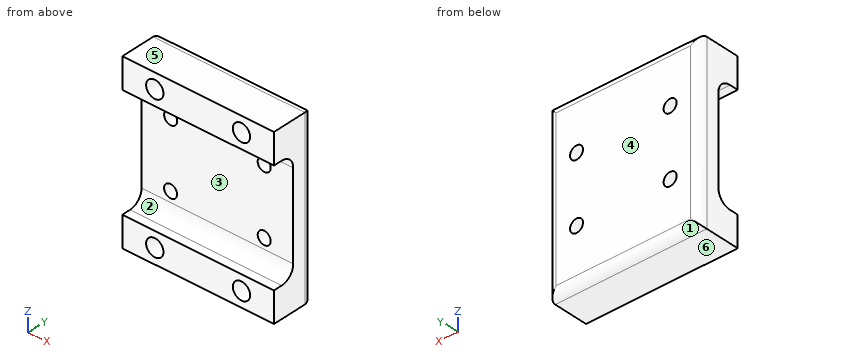
from build123d import *

# Parameters (mm, degrees)
SKETCH1_W            = 35
SKETCH1_H            = 40
BOSS_EXTRUDE1_DEPTH  = 5
SKETCH2_R            = 1.5
CUT_EXTRUDE1_DEPTH   = 5
SKETCH3_W            = 35
SKETCH3_H            = 7
BOSS_EXTRUDE2_DEPTH  = 5
SKETCH5_R            = 2
CUT_EXTRUDE3_DEPTH   = 8.5
FILLET2_R            = 3
FILLET3_R            = 2
FILLET2_OF_MIRROR2_R = 3


with BuildPart() as part:
    # Sketch1 → Boss-Extrude1 (new body)
    with BuildSketch(Plane(origin=(0, 0, 0), x_dir=(1, 0, 0), z_dir=(0, 1, 0))):
        Rectangle(SKETCH1_W, SKETCH1_H)
    extrude(amount=BOSS_EXTRUDE1_DEPTH)

    # Sketch2 → Cut-Extrude1 (cut)
    with BuildSketch(Plane(origin=(0, 5, 0), x_dir=(1, 0, 0), z_dir=(0, 1, 0))):
        with Locations(Location((-10.795, 7.62, 0), (0, 0, 270))):
            Circle(SKETCH2_R)
        with Locations(Location((10.795, 7.62, 0), (0, 0, 270))):
            Circle(SKETCH2_R)
        with Locations(Location((-10.795, -7.62, 0), (0, 0, 270))):
            Circle(SKETCH2_R)
        with Locations(Location((10.795, -7.62, 0), (0, 0, 270))):
            Circle(SKETCH2_R)
    extrude(amount=-CUT_EXTRUDE1_DEPTH, mode=Mode.SUBTRACT)

    # Sketch3 → Boss-Extrude2 (add)
    with BuildSketch(Plane.XZ):
        with Locations((0, 16.5)):
            Rectangle(SKETCH3_W, SKETCH3_H)
    boss_extrude2 = extrude(amount=BOSS_EXTRUDE2_DEPTH)

    # Sketch5 → Cut-Extrude3 (cut)
    with BuildSketch(Plane.XZ.offset(5)):
        with Locations(Location((-10, 16.5, 0), (0, 0, 270))):
            Circle(SKETCH5_R)
        with Locations(Location((10, 16.5, 0), (0, 0, 270))):
            Circle(SKETCH5_R)
    cut_extrude3 = extrude(amount=-CUT_EXTRUDE3_DEPTH, mode=Mode.SUBTRACT)

    # Fillet2
    fillet2_edges = [part.edges().sort_by_distance(p)[0] for p in [
        (0, 0, 13),
    ]]
    fillet(fillet2_edges, radius=FILLET2_R)

    # Fillet3
    fillet3_edges = [part.edges().sort_by_distance(p)[0] for p in [
        (17.5, 5, 0),
        (0, 5, -20),
        (-17.5, 5, 0),
        (0, 5, 20),
    ]]
    fillet(fillet3_edges, radius=FILLET3_R)

    # Mirror2: Boss-Extrude2, Cut-Extrude3 across plane
    add(boss_extrude2.mirror(Plane.XY))
    add(cut_extrude3.mirror(Plane.XY), mode=Mode.SUBTRACT)

    # Fillet2 of Mirror2
    fillet2_of_mirror2_edges = [part.edges().sort_by_distance(p)[0] for p in [
        (0, 0, -13),
    ]]
    fillet(fillet2_of_mirror2_edges, radius=FILLET2_OF_MIRROR2_R)


solid = part.part
Here's how the part is built. I have some questions about the finished solid (model axes, mm). Face numbers are marked on the shaded views. A direction names the side the tool comes from. Give positions to 0.01 mm unless a question says otherwise; leave off trailing zeros. Loops run counter-clockwise (first coordinate to the right, second up) from the corner with the lowest first, then second, coordinate; pieces in that order, holes last. Notation, with made-up numbers: (44.5, 62) -> (68.5, 62) arc R17 cw to (68.5, 82) -> close; hole circle Ø5 at (48.5, 3.25). An arc over 180 degrees is marked (long way). Answer as a JSON object with one key per item and string values. Group by question number.
Item 1: On a 3-axis mill with a long thin cutter (end or side, diameter ignored), from which of +Z, -Z, +X, -X, +Y, -Y can I reach the whole of each face in a straight line? I mean the marked faces 1 and 2. Say none if no direction works.
Item 2: I need wall thicknesses on L1, parallel to X at y = 2.15, z = -7.62 (3 decimals); L2, parallel to X at y = 2.75, z = -8; L3, parallel to Z at x = 4.5, y = -3.75. Which ranges of each line are inside material? Lowest first, please.
Item 3: Imagine slicing it at A-A on y = -1.75. Write out the boundary of the cut face in (x, z), then the cut area to 3 significant figures.
Item 4: Thinking about a two-plate mould opening in Z: for the marked faces 3, 4, 5 and 6, which applies, pulls with the +Z half, pulls with the -Z half, needs draft (parallel to the pull), parting line crosses it, or undercut?
Item 5: Imagine slicing it at B-B on z = -7.62. Write out the boundary of the cut face in (x, y) (3 decimals).
Item 6: Will these pins go through, and if not, where does the flat tip stop? pin 1 (3 mm diameter, centred on y = -0.5, z = -6.5, fed in from +X); pin 2 (3.5 mm diameter, centred on x = -10, z = -16.5, fed in from -Y); pin 3 (16 mm diameter, centred on x = -3.5, z = -3.5, fed in from -Y).
Item 7: Imagine slicing it at D-D on z = -2.5. Write out the boundary of the cut face in (x, y), then the cut area to 3 significant figures.
Item 8: Imagine slicing it at C-C on x = 10. Write out the boundary of the cut face in (y, z), then the cut area to 3 significant figures.
Answer list:
{
 "1": {"face 1": "-Z, +X, -X, +Y", "face 2": "+X, -X, -Y"},
 "2": {"L1": "x = -17.5 to -12.295, -9.295 to 9.295, 12.295 to 17.5", "L2": "x = -17.5 to -12.25, -9.34 to 9.34, 12.25 to 17.5", "L3": "z = -20 to -13, 13 to 20"},
 "3": {"outline": "(-17.5, -20) -> (17.5, -20) -> (17.5, -12.73) -> (-17.5, -12.73) -> close; (-17.5, 12.73) -> (17.5, 12.73) -> (17.5, 20) -> (-17.5, 20) -> close; hole circle Ø4 at (-10, -16.5); hole circle Ø4 at (-10, 16.5); hole circle Ø4 at (10, -16.5); hole circle Ø4 at (10, 16.5)", "area": "459 mm2"},
 "4": {"face 3": "undercut", "face 4": "needs draft", "face 5": "pulls with the +Z half", "face 6": "pulls with the -Z half"},
 "5": {"outline": "(-17.5, 0) -> (-12.295, 0) -> (-12.295, 5) -> (-15.5, 5) arc R2 ccw to (-17.5, 3) -> close; (-9.295, 0) -> (9.295, 0) -> (9.295, 5) -> (-9.295, 5) -> close; (12.295, 0) -> (17.5, 0) -> (17.5, 3) arc R2 ccw to (15.5, 5) -> (12.295, 5) -> close"},
 "6": {"pin 1": "stops at x = 17.5", "pin 2": "stops at y = 3.5", "pin 3": "stops at y = -0.4"},
 "7": {"outline": "(-17.5, 0) -> (17.5, 0) -> (17.5, 3) arc R2 ccw to (15.5, 5) -> (-15.5, 5) arc R2 ccw to (-17.5, 3) -> close", "area": "173 mm2"},
 "8": {"outline": "(-5, -20) -> (3, -20) arc R2 ccw to (5, -18) -> (5, -8.89) -> (0, -8.89) -> (0, -10) arc R3 cw to (-3, -13) -> (-5, -13) -> (-5, -14.5) -> (3.5, -14.5) -> (3.5, -18.5) -> (-5, -18.5) -> close; (-5, 13) -> (-3, 13) arc R3 cw to (0, 10) -> (0, 8.89) -> (5, 8.89) -> (5, 18) arc R2 ccw to (3, 20) -> (-5, 20) -> (-5, 18.5) -> (3.5, 18.5) -> (3.5, 14.5) -> (-5, 14.5) -> close; (0, -6.35) -> (5, -6.35) -> (5, 6.35) -> (0, 6.35) -> close", "area": "179 mm2"}
}
